Autodesk Inventor part; units mm, degrees
ref_plane "YZ Plane" through (0, 0, 0) normal (1, 0, 0) x (0, 1, 0)
ref_plane "XZ Plane" through (0, 0, 0) normal (0, 1, 0) x (-1, 0, 0)
ref_plane "XY Plane" through (0, 0, 0) normal (0, 0, 1) x (1, 0, 0)
sketch "Эскиз1" plane through (0, 0, 0) normal (0, 1, 0) x (-1, 0, 0)
  circle A0 centre (0, 0) radius 55
  line L0 (79.4555, 0) -> (-79.4555, 0)
  line L1 (0, -103.8803) -> (0, 88.3129)
  line L2 (38.15, -21.1) -> (-38.15, -21.1)
  line L3 (-38.15, -21.1) -> (-38.15, 21.1)
  line L4 (-38.15, 21.1) -> (38.15, 21.1)
  line L5 (38.15, 21.1) -> (38.15, -21.1)
  dimension "d0" = 110
  dimension "d60" = 76.3
  dimension "d61" = 42.2
extrude "Выдавливание1" add sketch "Эскиз1" along normal blind 1.6
sketch "Эскиз2" plane through (0, 0, 0) normal (0, -1, 0) x (1, 0, 0)
  circle A0 centre (0, 0) radius 55
  line L0 (0, -103.8803) -> (0, 88.3129)
  line L1 (-79.4555, 0) -> (79.4555, 0)
  circle A1 centre (0, 0) radius 50
  circle A2 centre (0, -50) radius 1.5
  circle A3 centre (50, 0) radius 1.5
  circle A4 centre (0, 50) radius 1.5
  circle A5 centre (-50, 0) radius 1.5
  circle A6 centre (35.3553, -35.3553) radius 1.5
  circle A7 centre (50, 0) radius 1.5
  circle A8 centre (35.3553, 35.3553) radius 1.5
  circle A9 centre (0, 50) radius 1.5
  circle A10 centre (-35.3553, 35.3553) radius 1.5
  circle A11 centre (-50, 0) radius 1.5
  circle A12 centre (-35.3553, -35.3553) radius 1.5
  line L2 (38.15, -20) -> (-39.85, -20)
  line L3 (-39.85, -20) -> (-39.85, 20)
  line L4 (-39.85, 20) -> (38.15, 20)
  line L5 (38.15, 20) -> (38.15, -20)
  line L6 (-27.5, 9.5) -> (27.5, 9.5)
  line L7 (27.5, 9.5) -> (27.5, -9.5)
  line L8 (27.5, -9.5) -> (-27.5, -9.5)
  line L9 (-27.5, -9.5) -> (-27.5, 9.5)
  circle A13 centre (27.5, 9.5) radius 1.5
  circle A14 centre (-27.5, 9.5) radius 1.5
  circle A15 centre (-27.5, -9.5) radius 1.5
  circle A16 centre (27.5, -9.5) radius 1.5
  circle A17 centre (0, -50) radius 1.5
  circle A18 centre (-10.5, -39) radius 1.5
  circle A19 centre (10.5, -39) radius 1.5
  point P0 (11.9394, -0.2)
  dimension "d22" = 3
  dimension "d23" = 3
  dimension "d25" = 3
  dimension "d26" = 3
  dimension "d30" = 360
  dimension "d62" = 78
  dimension "d63" = 40
  dimension "d70" = 110
  dimension "d71" = 55
  dimension "d72" = 19
  dimension "d73" = 3
  dimension "d74" = 3
  dimension "d75" = 3
  dimension "d76" = 3
extrude "Выдавливание2" cut sketch "Эскиз2" against normal blind 1.6 contours A3 A1 L1 | L1 A1 A3 | A4 A1 L0 | L0 A1 A4 | A2 A1 L0 | L0 A1 A2 | A1 A3 L1 | L1 A3 A1 | A5 A1 L1 | L1 A1 A5 | A1 A4 L0 | L0 A4 A1 | A1 A2 L0 | L0 A2 A1 | A8 A1 | A1 A8 | A6 A1 | A1 A6 | A1 A5 L1 | L1 A5 A1 | A10 A1 | A1 A10 | A12 A1 | A1 A12
extrude "Выдавливание5" [suppressed]
extrude "Выдавливание6" cut sketch "Эскиз2" against normal blind 10 contours A13 L6 L7 | L7 L6 A13 | A16 L8 L7 | L7 L8 A16 | A14 L9 L6 | L6 L9 A14 | A15 L9 L8 | L8 L9 A15 | A18 | A19
properties part number "pcbCase_last" material "Пластик АБС"
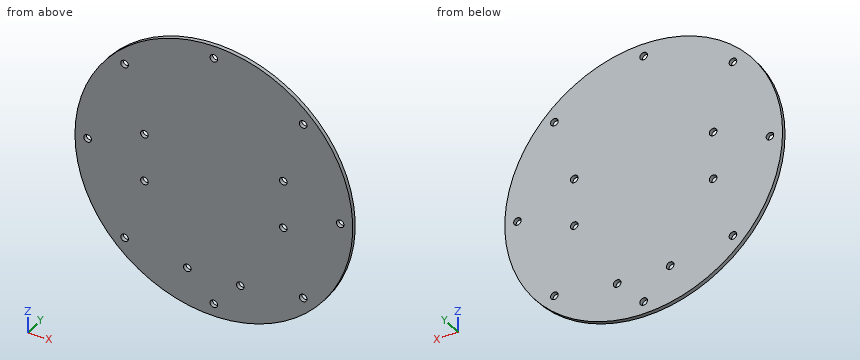
For this review, take the finished solid that the model builds, in its own axes (mm). Round coordinates to 2 decimals unless told otherwise and drop trailing zeros. Write each loop counter-clockwise with the first axis right and the second up, starting at its lowest first coordinate (ties: lowest second). Pieces come first, ordered by that corner, then holes. Notation, with made-up numbers: (0, 1) -> (29, 1) arc R18 cw to (29, 15) -> close; hole circle Ø8 at (15.5, 63.5). An arc over 180 degrees is marked (long way). One line per question, with ' | ' between items. Start each with the question number.
(1) Add section C-C, the plane x = 50. Write out the cut boundary in (y, z), plus the area to 3 significant figures.
(2) Add section A-A, the plane z = 50. Write out the cut boundary in (x, y), plus the area to 3 significant figures.
(3) Add section B-B, the plane y = 1.1. Give the number of separate pieces and of enclosed holes in the cut face, plus the area to 3 significant figures.
(4) Insertion check: P1, Ø1.8, axis at x = 27.5, z = -9.5, coming from the -Y side. The pin has a flat end and moves straight along its axis. Give the tip position at first contact, or say it passes through.
(5) Add section D-D, the plane z = -9.5. Write out the cut boundary in (x, y).
(6) For line 1 along Z through (x, y) = (0, 0.55); line 2 along Z through (x, y) = (-35, 0.9); line 3 along X through (y, z) = (1.1, -9.5), list the stretches that pass through material, from the lowest coordinate up. Write a range as from..to.
Answer list:
1) outline: (0, -22.91) -> (1.6, -22.91) -> (1.6, -1.5) -> (0, -1.5) -> close; (0, 1.5) -> (1.6, 1.5) -> (1.6, 22.91) -> (0, 22.91) -> close | area: 68.5 mm²
2) outline: (-22.91, 0) -> (-1.5, 0) -> (-1.5, 1.6) -> (-22.91, 1.6) -> close; (1.5, 0) -> (22.91, 0) -> (22.91, 1.6) -> (1.5, 1.6) -> close | area: 68.5 mm²
3) separate pieces: 1 | enclosed holes: 14 | area: 9,400 mm²
4) P1: through
5) outline: (-54.17, 0) -> (-29, 0) -> (-29, 1.6) -> (-54.17, 1.6) -> close; (-26, 0) -> (26, 0) -> (26, 1.6) -> (-26, 1.6) -> close; (29, 0) -> (54.17, 0) -> (54.17, 1.6) -> (29, 1.6) -> close
6) line 1: -55..-51.5, -48.5..48.5, 51.5..55 | line 2: -42.43..-36.81, -33.9..33.9, 36.81..42.43 | line 3: -54.17..-29, -26..26, 29..54.17
